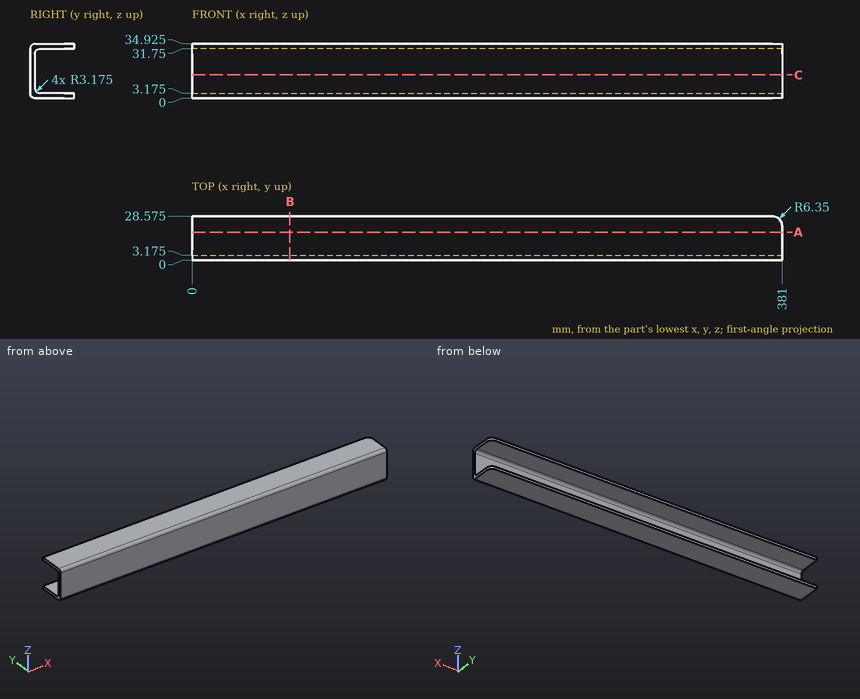
For this review, use the dimensioned drawing (mm, ordinates from the lowest corner) and the shaded views. Coordinates: 2 decimals unless noted, no trailing zeros. Order: outer loops, then holes, each group sorted by start corner. A loop starts at its lowest first (then second) coordinate and runs counter-clockwise, first axis right, second up. Notation, with made-up numbers: M 2,5.5 L 59,5.5 A18 cw 59,15.5 Z; hole C 28,56 d6. An arc over 180 degrees is marked long. Answer as a JSON object with one key per item and string values. Group by question number.
1) For pin 1 (11 mm diameter, centred on x = 215.5, z = 14, fed in from +Y) (3 decimals), flat-tipped, find the tip position at first contact; note if it passes through.
2) Add section A-A, the plane y = 18.25. Write out the cut boundary in (x, z) (3 decimals), then the cut area to 3 significant figures.
3) Add section C-C, the plane z = 15. Write out the cut boundary in (x, y) (3 decimals), then the cut area to 3 significant figures.
4) Add section B-B, the plane x = 63. Write out the cut boundary in (y, z) (3 decimals), then the cut area to 3 significant figures.
5) Wall thickness on L1, parallel to Z at x = 247.5, y = 7.5 (3 decimals); L2, parallel to Y at x = 322.5, z = 2.5 (3 decimals); L3, parallel to Y at x = 261, z = 17.5 (3 decimals): over which ranges is each line inside the solid? List them lowest first.
Computed values:
{
 "1": {"pin 1": "stops at y = 3.175"},
 "2": {"outline": "M 0,0 L 381,0 L 381,3.175 L 0,3.175 Z; M 0,31.75 L 381,31.75 L 381,34.925 L 0,34.925 Z", "area": "2,420 mm^2"},
 "3": {"outline": "M 0,0 L 381,0 L 381,3.175 L 0,3.175 Z", "area": "1,210 mm^2"},
 "4": {"outline": "M 0,3.175 A3.175 ccw 3.175,0 L 28.575,0 L 28.575,3.175 L 6.35,3.175 A3.175 cw 3.175,6.35 L 3.175,28.575 A3.175 cw 6.35,31.75 L 28.575,31.75 L 28.575,34.925 L 3.175,34.925 A3.175 ccw 0,31.75 Z", "area": "272 mm^2"},
 "5": {"L1": "z = 0 to 3.175, 31.75 to 34.925", "L2": "y = 0.073 to 28.575", "L3": "y = 0 to 3.175"}
}
